Geometry: final body of the model. Coordinates: model frame, mm. Round coordinates to 2 decimals unless told otherwise and drop trailing zeros. Loops run counter-clockwise (first coordinate to the right, second up) from the corner with the lowest first, then second, coordinate; pieces in that order, holes last. Notation, with made-up numbers: (35.5, 34.5) -> (85.5, 34.5) arc R13 ccw to (85.5, 52.5) -> close; hole circle Ø7 at (20, 74). An arc over 180 degrees is marked (long way). Answer in a Markdown table with one row per item.
```python
from build123d import *

# Parameters (mm, degrees)
SKETCH1_W           = 96
SKETCH1_H           = 300
SKETCH1_W_2         = 84
SKETCH1_H_2         = 92
BOSS_EXTRUDE1_DEPTH = 6
SKETCH2_R           = 1.3
CUT_EXTRUDE1_DEPTH  = 6
SKETCH4_R           = 1.3
CUT_EXTRUDE5_DEPTH  = 10
SKETCH3_R           = 1.3
CUT_EXTRUDE6_DEPTH  = 10


with BuildPart() as part:
    # Sketch1 → Boss-Extrude1 (new body)
    with BuildSketch(Plane.XY):
        Rectangle(SKETCH1_W, SKETCH1_H)
        with Locations((0, 98)):
            Rectangle(SKETCH1_W_2, SKETCH1_H_2, mode=Mode.SUBTRACT)
        with Locations((0, -98)):
            Rectangle(SKETCH1_W_2, SKETCH1_H_2, mode=Mode.SUBTRACT)
        Rectangle(SKETCH1_W_2, SKETCH1_H_2, mode=Mode.SUBTRACT)
    extrude(amount=BOSS_EXTRUDE1_DEPTH)

    # Sketch2 → Cut-Extrude1 (cut)
    with BuildSketch(Plane.XY.offset(6)):
        with Locations((-45, 147)):
            Circle(SKETCH2_R)
        with Locations((45, 147)):
            Circle(SKETCH2_R)
        with Locations((-45, -147)):
            Circle(SKETCH2_R)
        with Locations((45, -147)):
            Circle(SKETCH2_R)
    extrude(amount=-CUT_EXTRUDE1_DEPTH, mode=Mode.SUBTRACT)

    # Sketch4 → Cut-Extrude5 (cut)
    with BuildSketch(Plane(origin=(0, 150, 0), x_dir=(1, 0, 0), z_dir=(0, 1, 0))):
        with Locations(Location((-36, -3, 0), (0, 0, 270))):
            Circle(SKETCH4_R)
        with Locations(Location((36, -3, 0), (0, 0, 90))):
            Circle(SKETCH4_R)
    cut_extrude5 = extrude(amount=-CUT_EXTRUDE5_DEPTH, mode=Mode.SUBTRACT)

    # Mirror1: Cut-Extrude5 across plane
    add(cut_extrude5.mirror(Plane.ZX), mode=Mode.SUBTRACT)

    # Sketch3 → Cut-Extrude6 (cut)
    with BuildSketch(Plane.XY.offset(6)):
        with Locations((-45.000000047, 122)):
            Circle(SKETCH3_R)
        with Locations((-16.5, 147)):
            Circle(SKETCH3_R)
        with Locations(Location((16.5, 147, 0), (0, 0, 180))):
            Circle(SKETCH3_R)
        with Locations((-16.5, 49)):
            Circle(SKETCH3_R)
        with Locations(Location((16.5, 49, 0), (0, 0, 180))):
            Circle(SKETCH3_R)
        with Locations((-16.5, -49)):
            Circle(SKETCH3_R)
        with Locations(Location((16.5, -49, 0), (0, 0, 180))):
            Circle(SKETCH3_R)
        with Locations((-16.5, -147)):
            Circle(SKETCH3_R)
        with Locations(Location((16.5, -147, 0), (0, 0, 180))):
            Circle(SKETCH3_R)
        with Locations((-45.000000047, 21)):
            Circle(SKETCH3_R)
        with Locations((44.999999953, 122)):
            Circle(SKETCH3_R)
        with Locations((44.999999953, 77)):
            Circle(SKETCH3_R)
        with Locations((-45.000000047, 77)):
            Circle(SKETCH3_R)
        with Locations((44.999999953, 21)):
            Circle(SKETCH3_R)
        with Locations((44.999999953, -24)):
            Circle(SKETCH3_R)
        with Locations((-45.000000047, -24)):
            Circle(SKETCH3_R)
        with Locations((-45.000000047, -80)):
            Circle(SKETCH3_R)
        with Locations((44.999999953, -80)):
            Circle(SKETCH3_R)
        with Locations((44.999999953, -125)):
            Circle(SKETCH3_R)
        with Locations((-45.000000047, -125)):
            Circle(SKETCH3_R)
    extrude(amount=-CUT_EXTRUDE6_DEPTH, mode=Mode.SUBTRACT)


solid = part.part
```
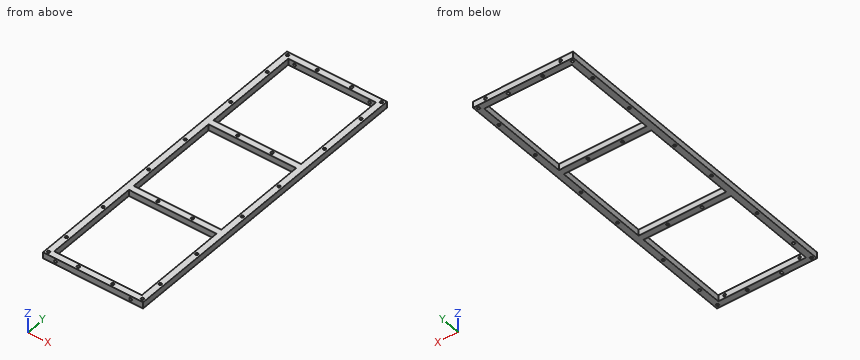
Item 1: Section query A-A, the plane y = 100.5. Output: boundary loops of the cut face in (x, z), and give its area (3 significant figures).
Ans:
| item | result |
|---|---|
| outline | (-48, 0) -> (-42, 0) -> (-42, 6) -> (-48, 6) -> close; (42, 0) -> (48, 0) -> (48, 6) -> (42, 6) -> close |
| area | 72.0 mm2 |
Item 2: Section query C-C, the plane z = 3. State how many separate pieces and enclosed holes the cut face has, and give its area (3 significant figures).
Ans:
| item | result |
|---|---|
| separate pieces | 3 |
| enclosed holes | 25 |
| area | 5,430 mm2 |
Item 3: Section query B-B, the plane x = 5.5. Output: boundary loops of the cut face in (y, z).
Ans:
| item | result |
|---|---|
| outline | (-150, 0) -> (-144, 0) -> (-144, 6) -> (-150, 6) -> close; (-52, 0) -> (-46, 0) -> (-46, 6) -> (-52, 6) -> close; (46, 0) -> (52, 0) -> (52, 6) -> (46, 6) -> close; (144, 0) -> (150, 0) -> (150, 6) -> (144, 6) -> close |
Item 4: Ray query, L1, parallel to Y at x = -25.5, z = 4.95; L2, parallel to X at y = -147, z = 1.3; L3, parallel to X at y = 124, z = 3.1. Return the intervals inside material, ascending.
Ans:
| item | result |
|---|---|
| L1 | -150 to -144, -52 to -46, 46 to 52, 144 to 150 |
| L2 | -48 to -46.3, -43.7 to -17.8, -15.2 to 15.2, 17.8 to 43.7, 46.3 to 48 |
| L3 | -48 to -42, 42 to 48 |
Item 5: First-contact query: P1, Ø4, axis at x = -45, y = -80, coming from the +Z side; P2, Ø2, axis at x = -36, z = 3, coming from the -Y side. Flat tips, straight axial feed; report the tip coordinate or a pass-through.
Ans:
| item | result |
|---|---|
| P1 | z = 6 |
| P2 | y = -52 |
